```python
from build123d import *

# Parameters (mm, degrees)
SKETCH1_R                        = 38.1
SKETCH1_R_2                      = 25.4
BOSS_EXTRUDE1_DEPTH              = 304.8
SKETCH2_R                        = 50.8
SKETCH2_R_2                      = 38.1
BOSS_EXTRUDE2_DEPTH              = 6.35
F_1_4_0_25_DIAMETER_HOLE1_D      = 6.35
SKETCH5_R                        = 28.6385
CUT_EXTRUDE1_DEPTH               = 6.477
SKETCH6_R                        = 30.2133
SKETCH6_R_2                      = 28.1051
CUT_EXTRUDE2_DEPTH               = 1.27
TAPPED_HOLE_FOR_6_32_HELICOIL1_D = 3.7338
CIRPATTERN1_COUNT                = 6


with BuildPart() as part:
    # Sketch1 → Boss-Extrude1 (new body)
    with BuildSketch(Plane(origin=(0, 0, 0), x_dir=(1, 0, 0), z_dir=(0, 1, 0))):
        with Locations(Location((0, 0, 0), (0, 0, 90))):
            Circle(SKETCH1_R)
        with Locations(Location((0, 0, 0), (0, 0, 90))):
            Circle(SKETCH1_R_2, mode=Mode.SUBTRACT)
    extrude(amount=BOSS_EXTRUDE1_DEPTH)

    # Sketch2 → Boss-Extrude2 (add)
    with BuildSketch(Plane(origin=(0, 0, 0), x_dir=(-1, 0, 0), z_dir=(0, -1, 0))):
        with Locations(Location((0, 0, 0), (0, 0, 90))):
            Circle(SKETCH2_R)
        with Locations(Location((0, 0, 0), (0, 0, 90))):
            Circle(SKETCH2_R_2, mode=Mode.SUBTRACT)
    extrude(amount=-BOSS_EXTRUDE2_DEPTH)

    # 1/4 (0.25) Diameter Hole1 (through all)
    with Locations(Plane(origin=(0, 0, 0), x_dir=(-1, 0, 0), z_dir=(0, -1, 0))):
        with Locations((0, -44.45), (-44.45, 0), (0, 44.45), (44.45, 0)):
            Hole(F_1_4_0_25_DIAMETER_HOLE1_D / 2)

    # Sketch5 → Cut-Extrude1 (cut)
    with BuildSketch(Plane(origin=(0, 0, 0), x_dir=(-1, 0, 0), z_dir=(0, -1, 0))):
        with Locations(Location((0, 0, 0), (0, 0, 90))):
            Circle(SKETCH5_R)
    extrude(amount=-CUT_EXTRUDE1_DEPTH, mode=Mode.SUBTRACT)

    # Sketch6 → Cut-Extrude2 (cut)
    with BuildSketch(Plane(origin=(0, 304.8, 0), x_dir=(1, 0, 0), z_dir=(0, 1, 0))):
        with Locations(Location((0, 0, 0), (0, 0, 270))):
            Circle(SKETCH6_R)
        with Locations(Location((0, 0, 0), (0, 0, 270))):
            Circle(SKETCH6_R_2, mode=Mode.SUBTRACT)
    extrude(amount=-CUT_EXTRUDE2_DEPTH, mode=Mode.SUBTRACT)

    # Tapped Hole for #6-32 Helicoil1 (through all)
    with Locations(Plane(origin=(0, 304.8, 0), x_dir=(1, 0, 0), z_dir=(0, 1, 0))):
        with Locations((0, 34.036)):
            tapped_hole_for_6_32_helicoil1 = Hole(TAPPED_HOLE_FOR_6_32_HELICOIL1_D / 2)

    # CirPattern1: Tapped Hole for #6-32 Helicoil1 ×6 about axis
    cirpattern1_axis = Axis((0, 0, 0), (0, 1, 0))
    for i in range(1, CIRPATTERN1_COUNT):
        add(tapped_hole_for_6_32_helicoil1.rotate(cirpattern1_axis, i * 360 / CIRPATTERN1_COUNT), mode=Mode.SUBTRACT)


solid = part.part
```
Source: CAD feature listing. Evaluate the final solid. Frame: model axes, mm. A direction names the side the tool comes from. Give positions to 0.01 mm unless a question says otherwise; leave off trailing zeros. Order: outer loops, then holes, each group sorted by start corner. A loop starts at its lowest first (then second) coordinate and runs counter-clockwise, first axis right, second up.
(1) Material intervals for line 1 along X through (y, z) = (283.5, 17.5); line 2 along Z through (x, y) = (-1.5, 242); line 3 along X through (y, z) = (130.5, -18), sorted ascending.
(2) Section query D-D (z = -44.45). Return the cut outline in (x, y) (3 decimals).
(3) Section query C-C (y = 268). Return the cut outline in (x, z).
(4) Access query for faces 1 (the face through (-22, 0, -22)), 2 (the face through (-10.969, 3.193, -26.455)), 3 (the face through (27.866, 304.174, -3.659)). Directions: +Z, -Z, +X, -X, +Y, -Y. A direction counts if a zero-diameter tool reaches every point of the face in a straight line with its end or side. Return the directions, or none.
(5) Section query A-A (z = 0). State how many separate pieces and enclosed holes the cut face has, plus the area to 3 significant figures.
(6) Pull-direction query (X, two-part tool) for faces 4 (the face through (-28.4, 304.8, -11.1)), 5 (the face through (-30.911, 3.131, 40.313)), 6 (the face through (41.28, 3.22, -0.14)); classes: +X half, -X half, draft (parallel to the pull), parting line (faces both ways), or undercut.
(7) Contact query for flat-ended pins moving along their axis: P1, Ø7.5, axis at x = 0, z = -44.45, coming from the +Y side; P2, Ø4, axis at y = 228.5, z = -6, coming from the -X side; P3, Ø8, axis at x = 13, y = 137.5, coming from the -Z side; P4, Ø5.5, axis at x = 0, z = 44.45, coming from the -Y side. Output: stop coordinate, or through.
(8) Section query B-B (x = 12). Return the cut outline in (y, z), plus the area to 3 significant figures.
Outcome:
1. line 1: x = -33.84 to -31.28, -27.67 to -18.41, 18.41 to 27.67, 31.28 to 33.84
1. line 2: z = -38.07 to -35.15, -32.92 to -25.36, 25.36 to 32.92, 35.15 to 38.07
1. line 3: x = -33.58 to -31.06, -27.89 to -17.92, 17.92 to 27.89, 31.06 to 33.58
2. outline: (-24.593, 0) - (-3.175, 0) - (-3.175, 6.35) - (-24.593, 6.35) - close; (3.175, 0) - (24.593, 0) - (24.593, 6.35) - (3.175, 6.35) - close
3. outline: circle Ø76.2 at (0, 0); hole circle Ø3.73 at (-29.48, -17.02); hole circle Ø3.73 at (-29.48, 17.02); hole circle Ø50.8 at (0, 0); hole circle Ø3.73 at (0, -34.04); hole circle Ø3.73 at (0, 34.04); hole circle Ø3.73 at (29.48, -17.02); hole circle Ø3.73 at (29.48, 17.02)
4. face 1: +Z, -Z, +X, -X, -Y
4. face 2: -Y
4. face 3: +Y
5. separate pieces: 4
5. enclosed holes: 0
5. area: 7,780 mm2
6. face 4: draft
6. face 5: parting line
6. face 6: undercut
7. P1: stops at y = 6.35
7. P2: stops at x = -37.89
7. P3: stops at z = -37.02
7. P4: passes through
8. outline: (0, -49.36) - (6.35, -49.36) - (6.35, -36.16) - (304.8, -36.16) - (304.8, -27.73) - (303.53, -27.73) - (303.53, -25.41) - (304.8, -25.41) - (304.8, -22.39) - (6.48, -22.39) - (6.48, -26) - (0, -26) - close; (0, 26) - (6.48, 26) - (6.48, 22.39) - (304.8, 22.39) - (304.8, 25.41) - (303.53, 25.41) - (303.53, 27.73) - (304.8, 27.73) - (304.8, 36.16) - (6.35, 36.16) - (6.35, 49.36) - (0, 49.36) - close
8. area: 8,510 mm2
